```python
from build123d import *

# Parameters (mm, degrees)
BOSS_EXTRUDE1_DEPTH = 5
SKETCH2_R           = 1
CUT_EXTRUDE1_DEPTH  = 5


with BuildPart() as part:
    # Sketch1 → Boss-Extrude1 (new body)
    with BuildSketch(Plane.XY):
        with BuildLine():
            Line((18.54, 0), (18.54, 3))
            Line((18.54, 3), (13.203469241, 3))
            ThreePointArc((13.203469241, 3), (0, 13.54), (-13.203469241, 3))
            Line((-13.203469241, 3), (-18.54, 3))
            Line((-18.54, 3), (-18.54, 0))
            Line((-18.54, 0), (-13.54, 0))
            Line((-13.54, 0), (-11.78, 0))
            ThreePointArc((-11.78, 0), (0, 11.78), (11.78, 0))
            Line((11.78, 0), (13.54, 0))
            Line((13.54, 0), (18.54, 0))
        make_face()
    extrude(amount=BOSS_EXTRUDE1_DEPTH)

    # Sketch2 → Cut-Extrude1 (cut)
    with BuildSketch(Plane(origin=(0, 3, 0), x_dir=(1, 0, 0), z_dir=(0, 1, 0))):
        with Locations(Location((-16.04, -2.5, 0), (0, 0, 270))):
            Circle(SKETCH2_R)
        with Locations(Location((16.04, -2.5, 0), (0, 0, 270))):
            Circle(SKETCH2_R)
    extrude(amount=-CUT_EXTRUDE1_DEPTH, mode=Mode.SUBTRACT)


solid = part.part
```
Design review of the part built by this model. Coordinates are the model's own, in mm. A direction names the side the tool comes from. Give positions to 0.01 mm unless a question says otherwise; leave off trailing zeros. Order: outer loops, then holes, each group sorted by start corner. A loop starts at its lowest first (then second) coordinate and runs counter-clockwise, first axis right, second up. Notation, with made-up numbers: (56, 38) -> (61, 38) arc R14 ccw to (61, 42) -> close; hole circle Ø5 at (80.5, -15.5). An arc over 180 degrees is marked (long way). Write each question's results on one line, items separated by ' | '. Start each with the question number.
Q1. Machinability: for faces 1 (the flat face through (16, 3, 1)), 2 (the cylindrical face through (16.716, 1.521, 1.763)), 3 (the flat face through (-16, 3, 1)), which of the approach directions +Z, -Z, +X, -X, +Y, -Y give a long, thin tool a straight path to every point of the face, cutting with its end or side? Answer none if there is none.
Q2. Mouldability with a two-part tool opening along X and no side actions: class faces 4 (the cylindrical face through (-17.016, 1.521, 2.283)), 5 (the cylindrical face through (-0.259, 11.777, 2.465)), 6 (the flat face through (-18.54, 2, 2)), 7 (the flat face through (0, 12, 0)) as +X half, -X half, draft (parallel to the pull), parting line (faces both ways), or undercut.
Q3. Add section B-B on y = 1.25. Give the boundary of the cut face in (x, z), and give its area (3 significant figures).
Q4. Add section D-D on y = 11. Give the boundary of the cut face in (x, z).
Q5. Add section C-C on x = 15.5. Give the boundary of the cut face in (y, z).
Q6. Wall thickness on L1, parallel to X at y = 1.1, z = 2.5; L2, parallel to X at y = 0.8, z = 2.5; L3, parallel to X at y = 3.75, z = 2.65: over which ranges is each line inside the solid? List them lowest first. Write a range as from..to.
Q7. Add section A-A on z = 2.5. Give the boundary of the cut face in (x, y).
Q8. For pin 1 (3 mm diameter, centred on y = 6.5, z = 3.5, fed in from +X); pin 2 (3 mm diameter, centred on x = 16.04, z = 2.5, fed in from +Y); pin 3 (1 mm diameter, centred on y = 10.5, z = 4.5, fed in from -X), all flat-tipped, find the tip position at first contact; note any pin that passes through.
Found:
1) face 1: +Z, -Z, +X, +Y | face 2: +Y, -Y | face 3: +Z, -Z, -X, +Y
2) face 4: undercut | face 5: undercut | face 6: -X half | face 7: draft
3) outline: (-18.54, 0) -> (-11.71, 0) -> (-11.71, 5) -> (-18.54, 5) -> close; (11.71, 0) -> (18.54, 0) -> (18.54, 5) -> (11.71, 5) -> close; hole circle Ø2 at (-16.04, 2.5); hole circle Ø2 at (16.04, 2.5) | area: 62.0 mm2
4) outline: (-7.9, 0) -> (-4.22, 0) -> (-4.22, 5) -> (-7.9, 5) -> close; (4.22, 0) -> (7.9, 0) -> (7.9, 5) -> (4.22, 5) -> close
5) outline: (0, 0) -> (3, 0) -> (3, 1.66) -> (0, 1.66) -> close; (0, 3.34) -> (3, 3.34) -> (3, 5) -> (0, 5) -> close
6) L1: x = -18.54..-17.04, -15.04..-11.73, 11.73..15.04, 17.04..18.54 | L2: x = -18.54..-17.04, -15.04..-11.75, 11.75..15.04, 17.04..18.54 | L3: x = -13.01..-11.17, 11.17..13.01
7) outline: (-18.54, 0) -> (-17.04, 0) -> (-17.04, 3) -> (-18.54, 3) -> close; (-15.04, 0) -> (-11.78, 0) arc R11.78 cw to (11.78, 0) -> (15.04, 0) -> (15.04, 3) -> (13.2, 3) arc R13.54 ccw to (-13.2, 3) -> (-15.04, 3) -> close; (17.04, 0) -> (18.54, 0) -> (18.54, 3) -> (17.04, 3) -> close
8) pin 1: stops at x = 12.58 | pin 2: stops at y = 3 | pin 3: stops at x = -9.13
